Check sheet for the modelled part. Datum: model origin and axes. Units: mm. A direction names the side the tool comes from. Round coordinates to 2 decimals unless told otherwise and drop trailing zeros. Order: outer loops, then holes, each group sorted by start corner. A loop starts at its lowest first (then second) coordinate and runs counter-clockwise, first axis right, second up. Notation, with made-up numbers: M -14,89 L -2,89 A11 cw -2,97 Z; hole C 19.25,-26 d7. An arc over 180 degrees is marked long. One line per item, written item: value. Start each with the question number.
(1) Depth check by flat-ended pin: pin 1 Ø4.5 at (x, z) = (-4, -27.25) entering from +Y; pin 2 Ø8 at (y, z) = (-28.5, -23) entering from -X; pin 3 Ø8.5 at (x, y) = (-18, -10.5) entering from -Z; pin 4 Ø4 at (x, y) = (-44, 0) entering from +Z. Enter the tip coordinate at first touch or a pass-through.
(2) Cross-section at C-C, the plane z = -27.25. Enter the section's corners in (x, y) (3 decimals).
(3) Release check for a two-part mould opening along X. For faces 1 (the face through (17.38, 0.44, 3.05)), 2 (the face through (21, -20, 3)), 3 (the face through (-14, 0.75, -4)) record: released by +X, released by -X, zero draft, split by the parting line, or undercut.
(4) Cross-section at B-B, the plane z = -5. Enter the section's corners in (x, y).
(5) Access from +Z, -Z, +X, -X, +Y, -Y to the whole of each face (thin tool, end or side, straight path). Record for faces 4 (the face through (-14, -2, 0)), 5 (the face through (-14, -8, -9)), 6 (the face through (16.669, -33.286, 3.054)), 7 (the face through (8, -28, -16)), 8 (the face through (-49, -20, 3)).
(6) Thickness scan on L1, parallel to X at y = -32, z = 2.3; L2, parallel to Y at x = -44, z = 3.1; L3, parallel to X at y = -7, z = 2. Record the ranges inside material, lowest first.
(7) Cross-section at D-D, the plane y = -26. Enter the section's corners in (x, z), and give its area (3 significant figures).
(8) Cross-section at A-A, the plane y = -12. Enter the section's corners in (x, z).
from build123d import *

# Parameters (mm, degrees)
SKETCH_1_W                     = 70
SKETCH_1_H                     = 43.75
EXTRUDE_1_DEPTH                = 6
EXTRUDE_2_DEPTH                = 15
CUT_EXTRUDE_1_DEPTH            = 13
EXTRUDE_4_DEPTH                = 6
EXTRUDE_5_DEPTH                = 44
FILLET_3_R                     = 1
FILLET_5_R                     = 4
FILLET_6_R                     = 1
FILLET_7_R                     = 5
HOLE_WIZARD_M2_5_1_D           = 2.9
HOLE_WIZARD_M2_5_1_CSINK_D     = 2.95
HOLE_WIZARD_M2_5_1_CSINK_ANGLE = 90
HOLE_WIZARD_M2_5_3_D           = 2.9
HOLE_WIZARD_M2_5_3_CSINK_D     = 2.95
HOLE_WIZARD_M2_5_3_CSINK_ANGLE = 90


with BuildPart() as part:
    # 草图1 → 凸台-拉伸1 (new body)
    with BuildSketch(Plane.XY):
        with Locations((-14, -16.875)):
            Rectangle(SKETCH_1_W, SKETCH_1_H)
    extrude(amount=EXTRUDE_1_DEPTH)

    # 草图2 → 凸台-拉伸2 (add)
    with BuildSketch(Plane.XY.offset(6)):
        Polygon((-13.907811237, 0.75), (8, 0.75), (8, -38.75), (-36, -38.75), (-36, 0.75), align=None)
    extrude(amount=-EXTRUDE_2_DEPTH)

    # 草图3 → 切除-拉伸1 (cut)
    with BuildSketch(Plane.XY.offset(6)):
        Polygon((-14, -2), (6, -2), (6, -38.75), (-34, -38.75), (-34, -2), align=None)
    extrude(amount=-CUT_EXTRUDE_1_DEPTH, mode=Mode.SUBTRACT)

    # 草图5 → 凸台-拉伸4 (add)
    with BuildSketch(Plane.XZ.offset(38.75)):
        with BuildLine():
            Line((-36, -9), (-36, -39))
            ThreePointArc((-36, -39), (-14, -46.202150475), (8, -39))
            Line((8, -39), (8, -9))
            Line((8, -9), (-36, -9))
        make_face()
    extrude(amount=-EXTRUDE_4_DEPTH)

    # 草图12 → 凸台-拉伸5 (add)
    with BuildSketch(Plane(origin=(8, 0, 0), x_dir=(0, 0, -1), z_dir=(1, 0, 0))):
        Polygon((9, -32.75), (22, -32.75), (9, -16), align=None)
    extrude(amount=-EXTRUDE_5_DEPTH)

    # 圆角3
    fillet_3_edges = [part.edges().sort_by_distance(p)[0] for p in [
        (-36, -35.75, -39),
        (-14, -32.75, -46.202150475),
        (8, -35.75, -39),
    ]]
    fillet(fillet_3_edges, radius=FILLET_3_R)

    # 圆角5
    fillet_5_edges = [part.edges().sort_by_distance(p)[0] for p in [
        (8, -19, 0),
        (-36, -19, 0),
    ]]
    fillet(fillet_5_edges, radius=FILLET_5_R)

    # 圆角6
    fillet_6_edges = [part.edges().sort_by_distance(p)[0] for p in [
        (6, -2, -0.5),
        (-34, -2, -0.5),
    ]]
    fillet(fillet_6_edges, radius=FILLET_6_R)

    # 圆角7
    fillet_7_edges = [part.edges().sort_by_distance(p)[0] for p in [
        (-49, 5, 3),
        (21, 5, 3),
    ]]
    fillet(fillet_7_edges, radius=FILLET_7_R)

    # M2.5 间隙孔1 (through all)
    with Locations(Plane(origin=(0, 0, 0), x_dir=(-1, 0, 0), z_dir=(0, 0, -1))):
        with Locations((-16, 0), (-16, -32), (44, -32), (44, 0)):
            CounterSinkHole(HOLE_WIZARD_M2_5_1_D / 2, HOLE_WIZARD_M2_5_1_CSINK_D / 2, counter_sink_angle=HOLE_WIZARD_M2_5_1_CSINK_ANGLE)

    # M2.5 间隙孔3 (through all)
    with Locations(Plane(origin=(0, -32.75, 0), x_dir=(1, 0, 0), z_dir=(0, 1, 0))):
        with Locations((-24, 27.25), (-4, 27.25)):
            CounterSinkHole(HOLE_WIZARD_M2_5_3_D / 2, HOLE_WIZARD_M2_5_3_CSINK_D / 2, counter_sink_angle=HOLE_WIZARD_M2_5_3_CSINK_ANGLE)


solid = part.part
Values found:
1. pin 1: y = -32.75
1. pin 2: x = -36
1. pin 3: z = -9
1. pin 4: z = 6
2. outline: M -36,-38.75 L -25.45,-38.75 L -25.45,-32.775 L -25.475,-32.75 L -36,-32.75 Z; M -22.55,-38.75 L -5.45,-38.75 L -5.45,-32.775 L -5.475,-32.75 L -22.525,-32.75 L -22.55,-32.775 Z; M -2.55,-38.75 L 8,-38.75 L 8,-32.75 L -2.525,-32.75 L -2.55,-32.775 Z
3. face 1: undercut
3. face 2: released by +X
3. face 3: zero draft
4. outline: M -36,-38.75 L -34,-38.75 L -34,-3 A1 cw -33,-2 L 5,-2 A1 cw 6,-3 L 6,-38.75 L 8,-38.75 L 8,0.75 L -36,0.75 Z
5. face 4: +Z, -Y
5. face 5: -Z, +X, -X, +Y
5. face 6: +Z, -Z
5. face 7: -Z, +X, +Y, -Y
5. face 8: +Z, -Z, -X, +Y, -Y
6. L1: -49 to -45.45, -42.55 to -34, 6 to 14.55, 17.45 to 21
6. L2: -38.75 to -33.45, -30.55 to -1.45, 1.45 to 5
6. L3: -49 to -34, 6 to 21
7. outline: M -49,0 L -40,0 A4 cw -36,-4 L -36,-16.76 L 8,-16.76 L 8,-4 A4 cw 12,0 L 21,0 L 21,6 L 6,6 L 6,-7 L -34,-7 L -34,6 L -49,6 Z
7. area: 644 mm^2
8. outline: M -49,0 L -40,0 A4 cw -36,-4 L -36,-9 L 8,-9 L 8,-4 A4 cw 12,0 L 21,0 L 21,6 L 6,6 L 6,-7 L -34,-7 L -34,6 L -49,6 Z
